Work out the finished part from the listing and answer in its coordinate system (mm). Coordinates: 2 decimals unless noted, no trailing zeros. Loops run counter-clockwise (first coordinate to the right, second up) from the corner with the lowest first, then second, coordinate; pieces in that order, holes last. Notation, with made-up numbers: M 87.25,-11.5 L 135.25,-11.5 A15 cw 135.25,5.5 Z; hole C 5.25,34.5 d5. An arc over 180 degrees is marked long. Write each question's results on one line, items separated by ' | '.
```python
from build123d import *

# Parameters (mm, degrees)
CROQUIS1_R              = 1.5
SALIENTE_EXTRUIR1_DEPTH = 2
REDONDEO1_R             = 5


with BuildPart() as part:
    # Croquis1 → Saliente-Extruir1 (new body)
    with BuildSketch(Plane(origin=(0, 0, 0), x_dir=(1, 0, 0), z_dir=(0, 1, 0))):
        Polygon((-13, 0), (-13, 5), (0, 5), (6.5, 5), (13, 2.5), (13, 0), (13, -2.5), (6.5, -5), (0, -5), (-13, -5), align=None)
        with Locations(Location((-9.5, 0, 0), (0, 0, 270))):
            Circle(CROQUIS1_R, mode=Mode.SUBTRACT)
    extrude(amount=SALIENTE_EXTRUIR1_DEPTH)

    # Redondeo1
    redondeo1_edges = [part.edges().sort_by_distance(p)[0] for p in [
        (-13, 1, 5),
        (-13, 1, -5),
    ]]
    fillet(redondeo1_edges, radius=REDONDEO1_R - 0.0001)  # a hair under: the kernel refuses the full size


solid = part.part
```
1) Find section C-C, the plane z = -0.5. Give the vertices of the cut face in (x, y), and give its area (3 significant figures).
Check result:
outline: M -12.97,0 L -10.91,0 L -10.91,2 L -12.97,2 Z; M -8.09,0 L 13,0 L 13,2 L -8.09,2 Z | area: 46.3 mm^2
2) Given pin 1 Ø2.5 at (x, z) = (-9.5, 0) entering from +Y, flat-ended and moving along its own axis, determine where the tip first touches the part or whether it passes through.
Check result:
pin 1: through
3) For a pull along X with two mould halves and no side action, classify faces 1 (the face through (9.8, 0.99, 3.73)), 2 (the face through (-11, 1, 0)), 3 (the face through (-1, 1, -5)), 4 (the face through (-12, 1, 3)) as released by +X, released by -X, zero draft, split by the parting line, or undercut.
Check result:
face 1: released by +X | face 2: undercut | face 3: zero draft | face 4: released by -X
4) Find section A-A, the plane x = -9.5. Give the vertices of the cut face in (y, z).
Check result:
outline: M 0,-4.77 L 2,-4.77 L 2,-1.5 L 0,-1.5 Z; M 0,1.5 L 2,1.5 L 2,4.77 L 0,4.77 Z
5) Straight lines are drawn through the part: probe 1 along X at (y, z) = (0.8, 0); probe 2 along Z at (x, y) = (-10.75, 0.4); probe 3 along Z at (x, y) = (-8.25, 0.6). For each, find the intervals that lie inside material, in ascending order. Write a range as [from, to].
Check result:
probe 1: [-13, -11], [-8, 13] | probe 2: [-4.18, -0.83], [0.83, 4.18] | probe 3: [-4.99, -0.83], [0.83, 4.99]
6) Find section D-D, the plane z = -3.5. Give the vertices of the cut face in (x, y).
Check result:
outline: M -11.57,0 L 10.4,0 L 10.4,2 L -11.57,2 Z
